For this review, take the finished solid that the model builds, in its own axes (mm). Coordinates: 2 decimals unless noted, no trailing zeros. Order: outer loops, then holes, each group sorted by start corner. A loop starts at its lowest first (then second) coordinate and runs counter-clockwise, first axis right, second up. Notation, with made-up numbers: (-37.5, 23) - (-4.5, 23) arc R18 cw to (-4.5, 32) - close; hole circle Ø7 at (49.25, 32). An arc over 180 degrees is marked (long way). One line per item, written item: value. Start each with the question number.
(1) Consider section A-A on x = -17.5. Write out the cut boundary in (y, z), then the cut area to 3 significant figures.
(2) To check wall thickness, follow line 1 along Y through (x, z) = (-28.5, 0.7); line 2 along X through (y, z) = (-30, 0.55); line 3 along X through (y, z) = (-30.5, 0.65). State the ranges of each line that lie inside material, in increasing order.
(3) Clearance check with flat-ended pins moving along their axes: pin 1 (0.5 mm diameter, centred on x = 2.5, z = 0.5, fed in from +Y); pin 2 (2.5 mm diameter, centred on x = -35, y = -15, fed in from -Z); pin 3 (0.5 mm diameter, centred on x = 18, z = 0.5, fed in from -Y). State where each tip first meets the part, or that it passes through.
(4) Consider section D-D on y = -8. Write out the cut boundary in (x, z), then the cut area to 3 significant figures.
(5) Consider section B-B on y = -19.5. Write out the cut boundary in (x, z).
(6) Consider section C-C on x = -35. Write out the cut boundary in (y, z).
```python
from build123d import *

# Parameters (mm, degrees)
MODEL_R         = 4.2
MODEL_R_2       = 1.5
EXTRUDE_1_DEPTH = 1


with BuildPart() as part:
    # Model → Бобышка-Вытянуть1 (new body)
    with BuildSketch(Plane.XY):
        with BuildLine():
            ThreePointArc((-40, 11), (-39.707106781, 10.292893219), (-39, 10))
            Line((-39, 10), (-30.5, 10))
            ThreePointArc((-30.5, 10), (-29.792893219, 9.707106781), (-29.5, 9))
            Line((-29.5, 9), (-29.5, 0))
            Line((-29.5, 0), (-29.5, -9))
            ThreePointArc((-29.5, -9), (-29.792893219, -9.707106781), (-30.5, -10))
            Line((-30.5, -10), (-39, -10))
            ThreePointArc((-39, -10), (-39.707106781, -10.292893219), (-40, -11))
            Line((-40, -11), (-40, -15))
            Line((-40, -15), (-40, -19))
            Line((-40, -19), (-40, -31.96122651))
            ThreePointArc((-40, -31.96122651), (-31.378483084, -39.978850181), (-24.006941008, -30.798806025))
            ThreePointArc((-24.006941008, -30.798806025), (-23.966641223, -30.339501194), (-23.724557848, -29.947097523))
            Line((-23.724557848, -29.947097523), (-20.270353544, -26.492893219))
            ThreePointArc((-20.270353544, -26.492893219), (-19.945930196, -26.276120467), (-19.563246763, -26.2))
            Line((-19.563246763, -26.2), (-16.149033201, -26.2))
            ThreePointArc((-16.149033201, -26.2), (-15.766349768, -26.123879533), (-15.44192642, -25.907106781))
            Line((-15.44192642, -25.907106781), (-6.827712857, -17.292893219))
            ThreePointArc((-6.827712857, -17.292893219), (-6.503289508, -17.076120467), (-6.120606076, -17))
            Line((-6.120606076, -17), (0, -17))
            Line((0, -17), (6.120606076, -17))
            ThreePointArc((6.120606076, -17), (6.503289508, -17.076120467), (6.827712857, -17.292893219))
            Line((6.827712857, -17.292893219), (15.44192642, -25.907106781))
            ThreePointArc((15.44192642, -25.907106781), (15.766349768, -26.123879533), (16.149033201, -26.2))
            Line((16.149033201, -26.2), (19.563246763, -26.2))
            ThreePointArc((19.563246763, -26.2), (19.945930196, -26.276120467), (20.270353544, -26.492893219))
            Line((20.270353544, -26.492893219), (23.724557848, -29.947097523))
            ThreePointArc((23.724557848, -29.947097523), (23.966641223, -30.339501194), (24.006941008, -30.798806025))
            ThreePointArc((24.006941008, -30.798806025), (31.378483084, -39.978850181), (40, -31.96122651))
            Line((40, -31.96122651), (40, -19))
            Line((40, -19), (40, -15))
            Line((40, -15), (40, -11))
            ThreePointArc((40, -11), (39.707106781, -10.292893219), (39, -10))
            Line((39, -10), (30.5, -10))
            ThreePointArc((30.5, -10), (29.792893219, -9.707106781), (29.5, -9))
            Line((29.5, -9), (29.5, 0))
            Line((29.5, 0), (29.5, 9))
            ThreePointArc((29.5, 9), (29.792893219, 9.707106781), (30.5, 10))
            Line((30.5, 10), (39, 10))
            ThreePointArc((39, 10), (39.707106781, 10.292893219), (40, 11))
            Line((40, 11), (40, 15))
            Line((40, 15), (40, 19))
            Line((40, 19), (40, 31.96122651))
            ThreePointArc((40, 31.96122651), (31.378483084, 39.978850181), (24.006941008, 30.798806025))
            ThreePointArc((24.006941008, 30.798806025), (23.966641223, 30.339501194), (23.724557848, 29.947097523))
            Line((23.724557848, 29.947097523), (20.270353544, 26.492893219))
            ThreePointArc((20.270353544, 26.492893219), (19.945930196, 26.276120467), (19.563246763, 26.2))
            Line((19.563246763, 26.2), (16.149033201, 26.2))
            ThreePointArc((16.149033201, 26.2), (15.766349768, 26.123879533), (15.44192642, 25.907106781))
            Line((15.44192642, 25.907106781), (6.827712857, 17.292893219))
            ThreePointArc((6.827712857, 17.292893219), (6.503289508, 17.076120467), (6.120606076, 17))
            Line((6.120606076, 17), (0, 17))
            Line((0, 17), (-6.120606076, 17))
            ThreePointArc((-6.120606076, 17), (-6.503289508, 17.076120467), (-6.827712857, 17.292893219))
            Line((-6.827712857, 17.292893219), (-15.44192642, 25.907106781))
            ThreePointArc((-15.44192642, 25.907106781), (-15.766349768, 26.123879533), (-16.149033201, 26.2))
            Line((-16.149033201, 26.2), (-19.563246763, 26.2))
            ThreePointArc((-19.563246763, 26.2), (-19.945930196, 26.276120467), (-20.270353544, 26.492893219))
            Line((-20.270353544, 26.492893219), (-23.724557848, 29.947097523))
            ThreePointArc((-23.724557848, 29.947097523), (-23.966641223, 30.339501194), (-24.006941008, 30.798806025))
            ThreePointArc((-24.006941008, 30.798806025), (-31.378483084, 39.978850181), (-40, 31.96122651))
            Line((-40, 31.96122651), (-40, 19))
            Line((-40, 19), (-40, 15))
            Line((-40, 15), (-40, 11))
        make_face()
        with Locations((-31.96122651, -31.96122651)):
            Circle(MODEL_R, mode=Mode.SUBTRACT)
        with Locations((-35, -15)):
            Circle(MODEL_R_2, mode=Mode.SUBTRACT)
        with BuildLine():
            ThreePointArc((-23.5, -4), (-23.207106781, -3.292893219), (-22.5, -3))
            Line((-22.5, -3), (-9.656854249, -3))
            ThreePointArc((-9.656854249, -3), (-8.732974717, -3.617316568), (-8.949747468, -4.707106781))
            Line((-8.949747468, -4.707106781), (-21.792893219, -17.550252532))
            ThreePointArc((-21.792893219, -17.550252532), (-22.882683432, -17.767025283), (-23.5, -16.843145751))
            Line((-23.5, -16.843145751), (-23.5, -6.777502295))
            Line((-23.5, -6.777502295), (-23.5, -4))
        make_face(mode=Mode.SUBTRACT)
        with Locations((31.96122651, -31.96122651)):
            Circle(MODEL_R, mode=Mode.SUBTRACT)
        with BuildLine():
            Line((9.656854249, -3), (22.5, -3))
            ThreePointArc((22.5, -3), (23.207106781, -3.292893219), (23.5, -4))
            Line((23.5, -4), (23.5, -6.777502295))
            Line((23.5, -6.777502295), (23.5, -16.843145751))
            ThreePointArc((23.5, -16.843145751), (22.882683432, -17.767025283), (21.792893219, -17.550252532))
            Line((21.792893219, -17.550252532), (8.949747468, -4.707106781))
            ThreePointArc((8.949747468, -4.707106781), (8.732974717, -3.617316568), (9.656854249, -3))
        make_face(mode=Mode.SUBTRACT)
        with BuildLine():
            Line((7.343145751, -14), (0, -14))
            Line((0, -14), (-7.343145751, -14))
            ThreePointArc((-7.343145751, -14), (-8.267025283, -13.382683432), (-8.050252532, -12.292893219))
            Line((-8.050252532, -12.292893219), (-0.707106781, -4.949747468))
            ThreePointArc((-0.707106781, -4.949747468), (-0.382683432, -4.732974717), (0, -4.656854249))
            ThreePointArc((0, -4.656854249), (0.382683432, -4.732974717), (0.707106781, -4.949747468))
            Line((0.707106781, -4.949747468), (8.050252532, -12.292893219))
            ThreePointArc((8.050252532, -12.292893219), (8.267025283, -13.382683432), (7.343145751, -14))
        make_face(mode=Mode.SUBTRACT)
        with Locations((35, -15)):
            Circle(MODEL_R_2, mode=Mode.SUBTRACT)
        with Locations((-35, 15)):
            Circle(MODEL_R_2, mode=Mode.SUBTRACT)
        with BuildLine():
            Line((-7.343145751, 14), (0, 14))
            Line((0, 14), (7.343145751, 14))
            ThreePointArc((7.343145751, 14), (8.267025283, 13.382683432), (8.050252532, 12.292893219))
            Line((8.050252532, 12.292893219), (0.707106781, 4.949747468))
            ThreePointArc((0.707106781, 4.949747468), (0.382683432, 4.732974717), (0, 4.656854249))
            ThreePointArc((0, 4.656854249), (-0.382683432, 4.732974717), (-0.707106781, 4.949747468))
            Line((-0.707106781, 4.949747468), (-8.050252532, 12.292893219))
            ThreePointArc((-8.050252532, 12.292893219), (-8.267025283, 13.382683432), (-7.343145751, 14))
        make_face(mode=Mode.SUBTRACT)
        with BuildLine():
            Line((-9.656854249, 3), (-22.5, 3))
            ThreePointArc((-22.5, 3), (-23.207106781, 3.292893219), (-23.5, 4))
            Line((-23.5, 4), (-23.5, 6.777502295))
            Line((-23.5, 6.777502295), (-23.5, 16.843145751))
            ThreePointArc((-23.5, 16.843145751), (-22.882683432, 17.767025283), (-21.792893219, 17.550252532))
            Line((-21.792893219, 17.550252532), (-8.949747468, 4.707106781))
            ThreePointArc((-8.949747468, 4.707106781), (-8.732974717, 3.617316568), (-9.656854249, 3))
        make_face(mode=Mode.SUBTRACT)
        with Locations((-31.96122651, 31.96122651)):
            Circle(MODEL_R, mode=Mode.SUBTRACT)
        with BuildLine():
            ThreePointArc((23.5, 4), (23.207106781, 3.292893219), (22.5, 3))
            Line((22.5, 3), (9.656854249, 3))
            ThreePointArc((9.656854249, 3), (8.732974717, 3.617316568), (8.949747468, 4.707106781))
            Line((8.949747468, 4.707106781), (21.792893219, 17.550252532))
            ThreePointArc((21.792893219, 17.550252532), (22.882683432, 17.767025283), (23.5, 16.843145751))
            Line((23.5, 16.843145751), (23.5, 6.777502295))
            Line((23.5, 6.777502295), (23.5, 4))
        make_face(mode=Mode.SUBTRACT)
        with Locations((35, 15)):
            Circle(MODEL_R_2, mode=Mode.SUBTRACT)
        with Locations((31.96122651, 31.96122651)):
            Circle(MODEL_R, mode=Mode.SUBTRACT)
    extrude(amount=EXTRUDE_1_DEPTH)


solid = part.part
```
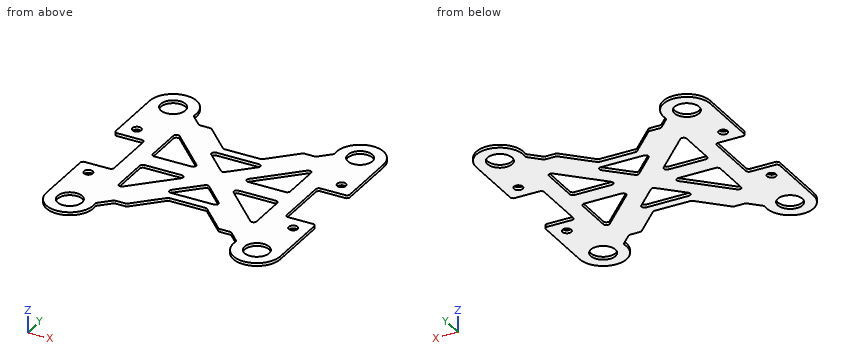
Geometry check:
1. outline: (-26.2, 0) - (-13.26, 0) - (-13.26, 1) - (-26.2, 1) - close; (-3, 0) - (3, 0) - (3, 1) - (-3, 1) - close; (13.26, 0) - (26.2, 0) - (26.2, 1) - (13.26, 1) - close
1. area: 31.9 mm^2
2. line 1: y = -39.22 to -34.34, -29.58 to 29.58, 34.34 to 39.22
2. line 2: x = -40 to -35.68, -28.25 to -23.77, 23.77 to 28.25, 35.68 to 40
2. line 3: x = -40 to -35.9, -28.02 to -24.01, 24.01 to 28.02, 35.9 to 40
3. pin 1: stops at y = 17
3. pin 2: passes through
3. pin 3: stops at y = -26.2
4. outline: (-29.5, 0) - (-23.5, 0) - (-23.5, 1) - (-29.5, 1) - close; (-12.24, 0) - (-3.76, 0) - (-3.76, 1) - (-12.24, 1) - close; (3.76, 0) - (12.24, 0) - (12.24, 1) - (3.76, 1) - close; (23.5, 0) - (29.5, 0) - (29.5, 1) - (23.5, 1) - close
4. area: 29.0 mm^2
5. outline: (-40, 0) - (-9.03, 0) - (-9.03, 1) - (-40, 1) - close; (9.03, 0) - (40, 0) - (40, 1) - (9.03, 1) - close
6. outline: (-39.4, 0) - (-34.86, 0) - (-34.86, 1) - (-39.4, 1) - close; (-29.06, 0) - (-16.5, 0) - (-16.5, 1) - (-29.06, 1) - close; (-13.5, 0) - (-10, 0) - (-10, 1) - (-13.5, 1) - close; (10, 0) - (13.5, 0) - (13.5, 1) - (10, 1) - close; (16.5, 0) - (29.06, 0) - (29.06, 1) - (16.5, 1) - close; (34.86, 0) - (39.4, 0) - (39.4, 1) - (34.86, 1) - close
